Answer from the drawing. Dimensions are ordinates in mm from the lowest x, y and z of the part. A direction names the side the tool comes from. Coordinates: 2 decimals unless noted, no trailing zeros. Order: outer loops, then holes, each group sorted by start corner. A loop starts at its lowest first (then second) coordinate and runs counter-clockwise, first axis right, second up.
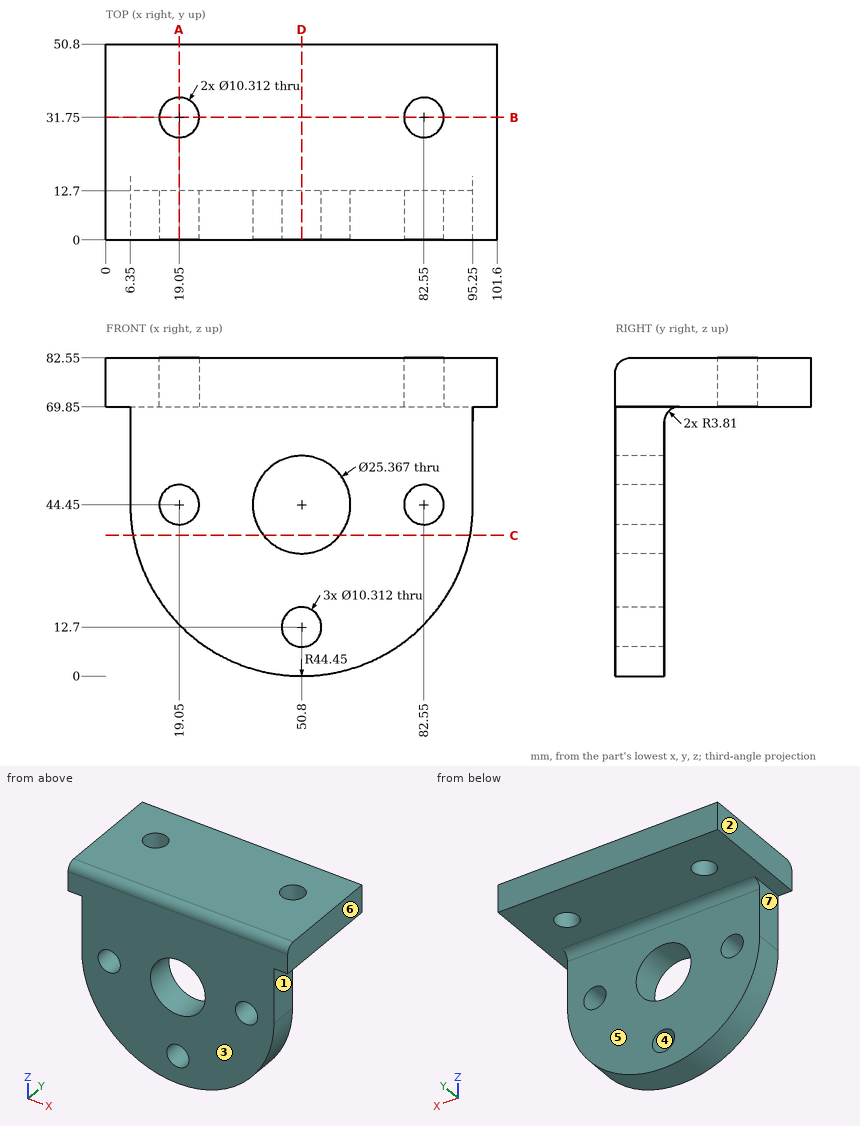
1) Consider L1, parallel to X at y = 6, z = 44 (1 decimal); L2, parallel to Y at x = 19, z = 76; L3, parallel to Y at x = 43, z = 10. Determine where each line is inside the solid, lowest interval first.
2) Section B-B (y = 31.75) is taken. Give the vertices of the cut face in (x, z).
3) Each of these flat-tipped pins is pushed along its axis until it touches: P1, Ø1, axis at x = 31.5, z = 40.5, coming from the +Y side; P2, Ø1.5, axis at y = 7.5, z = 40.5, coming from the +X side (1 decimal); P3, Ø8, axis at y = 10, z = 64.5, coming from the +X side. Where does it stop, or does it pass through?
4) Determine the mould class of the marked faces 1, 2, 3 and 4 for opening direction X: released by +X, released by -X, zero draft, split by the parting line, or undercut.
5) Section C-C (z = 36.5) is taken. Give the vertices of the cut face in (x, y), then the cut area to 3 significant figures.
6) A tool of negligible diameter and unlimited length cuts with its end or side. For the marked faces 5, 6 and 7, from which of +Z, -Z, +X, -X, +Y, -Y can it reach the whole face along a straight path? Write none if from no direction.
7) Section D-D (x = 50.8) is taken. Give the vertices of the cut face in (y, z).
8) Section A-A (x = 19.05) is taken. Give the vertices of the cut face in (y, z).
Filled sheet:
1. L1: x = 6.4 to 13.9, 24.2 to 38.1, 63.5 to 77.4, 87.7 to 95.2
1. L2: y = 0 to 26.59, 36.91 to 50.8
1. L3: y = 0 to 12.7
2. outline: (0, 69.85) - (13.89, 69.85) - (13.89, 82.55) - (0, 82.55) - close; (24.21, 69.85) - (77.39, 69.85) - (77.39, 82.55) - (24.21, 82.55) - close; (87.71, 69.85) - (101.6, 69.85) - (101.6, 82.55) - (87.71, 82.55) - close
3. P1: stops at y = 12.7
3. P2: stops at x = 95.1
3. P3: stops at x = 95.25
4. face 1: released by +X
4. face 2: released by -X
4. face 3: zero draft
4. face 4: undercut
5. outline: (7.07, 0) - (40.92, 0) - (40.92, 12.7) - (7.07, 12.7) - close; (60.68, 0) - (94.53, 0) - (94.53, 12.7) - (60.68, 12.7) - close
5. area: 860 mm2
6. face 5: -Z, +X, -X, +Y
6. face 6: +Z, -Z, +X, +Y, -Y
6. face 7: -Z, -X, +Y, -Y
7. outline: (0, 0) - (12.7, 0) - (12.7, 7.54) - (0, 7.54) - close; (0, 17.86) - (12.7, 17.86) - (12.7, 31.77) - (0, 31.77) - close; (0, 57.13) - (12.7, 57.13) - (12.7, 66.04) arc R3.81 cw to (16.51, 69.85) - (50.8, 69.85) - (50.8, 82.55) - (3.81, 82.55) arc R3.81 ccw to (0, 78.74) - close
8. outline: (0, 13.34) - (12.7, 13.34) - (12.7, 39.29) - (0, 39.29) - close; (0, 49.61) - (12.7, 49.61) - (12.7, 66.04) arc R3.81 cw to (16.51, 69.85) - (26.59, 69.85) - (26.59, 82.55) - (3.81, 82.55) arc R3.81 ccw to (0, 78.74) - close; (36.91, 69.85) - (50.8, 69.85) - (50.8, 82.55) - (36.91, 82.55) - close
